```python
from build123d import *

# Parameters (mm, degrees)
F0_R          = 0.79375
F1_DEPTH      = 5.334
F3_DEPTH      = 5.334
F4_R          = 0.127
F5_W          = 2.54
F5_H          = 2.8669180299
F6_DEPTH      = 3.0408234879
F6_DEPTH_BACK = 0.8715074616
F7_SIZE       = 2.032


with BuildPart() as f1:
    # F0 (on Front) → F1 (new body)
    with BuildSketch(Plane.XZ):
        with BuildLine():
            ThreePointArc((-1.5158234879, 0.1576551724), (0, -1.524), (1.5158234879, 0.1576551724))
            Line((1.5158234879, 0.1576551724), (0.757911744, 7.4448275862))
            ThreePointArc((0.757911744, 7.4448275862), (0, 8.128), (-0.757911744, 7.4448275862))
            Line((-0.757911744, 7.4448275862), (-1.5158234879, 0.1576551724))
        make_face()
        Circle(F0_R, mode=Mode.SUBTRACT)
    extrude(amount=F1_DEPTH)

    # F2 (on face) → F3 (join, through all)
    with BuildSketch(Plane.XZ.offset(5.334)):
        Polygon((1.5158234879, 2.6129180299), (1.2631934914, 2.586642922), (1.5158234879, 0.1576551724), align=None)
        with BuildLine():
            Line((2.62023831, 4.4970114676), (0.6525069605, 7.7595462699))
            ThreePointArc((0.6525069605, 7.7595462699), (0.7225525537, 7.6079954691), (0.757911744, 7.4448275862))
            Line((0.757911744, 7.4448275862), (0.9662072397, 5.4421073456))
            Line((0.9662072397, 5.4421073456), (2.62023831, 4.4970114676))
        make_face()
    extrude(amount=-F3_DEPTH)

    # F4
    f4_edges = [f1.edges().sort_by_distance(p)[0] for p in [
        (2.620238, -2.667, 4.497011),
        (0.966207, -2.667, 5.442107),
    ]]
    fillet(f4_edges, radius=F4_R)

    # F5 (on face) → F6 (cut, two sides)
    with BuildSketch(Plane.YZ.offset(1.5158234879)) as f6_sk:
        with Locations((-2.667, -0.090540985)):
            Rectangle(F5_W, F5_H)
    extrude(amount=-F6_DEPTH, mode=Mode.SUBTRACT)
    extrude(f6_sk.sketch, amount=F6_DEPTH_BACK, mode=Mode.SUBTRACT)

    # F7
    f7_edges = [f1.edges().sort_by_distance(p)[0] for p in [
        (-1.392549, -2.667, 1.342918),
    ]]
    chamfer(f7_edges, length=F7_SIZE)


solid = f1.part
```
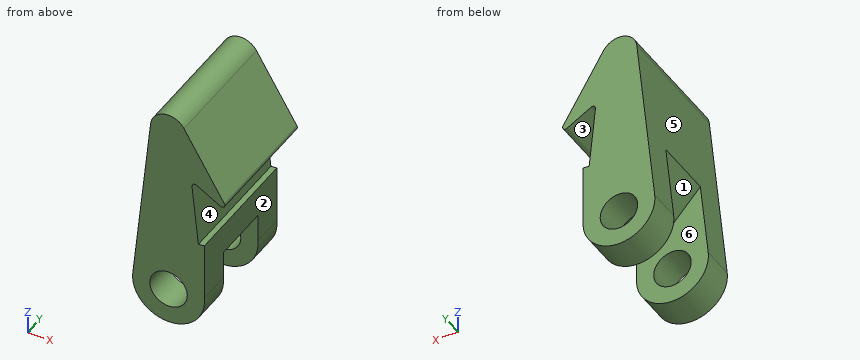
The model under review builds one solid part; all positions refer to its coordinate system, in mm. Face numbers are marked on the shaded views. A direction names the side the tool comes from. Coordinates: 2 decimals unless noted, no trailing zeros. Write each loop counter-clockwise with the first axis right and the second up, starting at its lowest first coordinate (ties: lowest second). Pieces come first, ordered by that corner, then holes. Notation, with made-up numbers: (28.25, 0) - (41.25, 0) arc R34 cw to (41.25, 37) - close; hole circle Ø2 at (89.25, -23.75). An arc over 180 degrees is marked (long way). Answer in a Markdown table with one row per item. Add a question column.
Q1. Consider section A-A on z = 0. Give the boundary of the cut face in (x, y).
Q2. For the marked faces 1, 2 and 3, list the 3-axis set-ups (+Z, -Z, +X, -X, +Y, -Y) from which the entire face can be reached by the end or side of a thin tool; tool diameter is ignored.
Q3. Consider section D-D on z = 1. Give the boundary of the cut face in (x, y), then the cut area to 3 significant figures.
Q4. Consider section B-B on x = 0.25. Give the boundary of the cut face in (y, z).
Q5. To check wall thickness, follow line 1 along X through (y, z) = (-0.6, 0); line 2 along Y through (x, z) = (1.4, 0.75); line 3 along Z through (x, y) = (2.2, -0.85). State the ranges of each line that lie inside material, in increasing order. Write a range as from..to.
Q6. Draft analysis for pull direction Z (two halves, no side actions). For the marked faces 4, 5 and 6, state which applies: +Z half, -Z half, draft (parallel to the pull), parting line (faces both ways), or undercut.
Q7. Clearance check with flat-ended pins moving along their axes: pin 1 (1 mm diameter, centred on x = 1, y = -2, fed in from -Z); pin 2 (2.5 mm diameter, centred on y = -3.5, z = 2, fed in from +X). State where each tip first meets the part, or that it passes through.
Answers below:
| question | item | result |
|---|---|---|
| 1 | outline | (-1.52, -5.33) - (-0.79, -5.33) - (-0.79, -3.94) - (-1.52, -3.94) - close; (-1.52, -1.4) - (-0.79, -1.4) - (-0.79, 0) - (-1.52, 0) - close; (0.79, -5.33) - (1.52, -5.33) - (1.52, -3.94) - (0.79, -3.94) - close; (0.79, -1.4) - (1.52, -1.4) - (1.52, 0) - (0.79, 0) - close |
| 2 | face 1 | -Z, -X |
| 2 | face 2 | +X, +Y, -Y |
| 2 | face 3 | +Y, -Y |
| 3 | outline | (-1.43, -5.33) - (1.52, -5.33) - (1.52, -3.94) - (-1.43, -3.94) - close; (-1.43, -1.4) - (1.52, -1.4) - (1.52, 0) - (-1.43, 0) - close |
| 3 | area | 8.23 mm² |
| 4 | outline | (-5.33, -1.5) - (-3.94, -1.5) - (-3.94, -0.75) - (-5.33, -0.75) - close; (-5.33, 0.75) - (-3.94, 0.75) - (-3.94, 1.77) - (-1.4, 1.77) - (-1.4, 0.75) - (0, 0.75) - (0, 8.09) - (-5.33, 8.09) - close; (-1.4, -1.5) - (0, -1.5) - (0, -0.75) - (-1.4, -0.75) - close |
| 5 | line 1 | -1.52..-0.79, 0.79..1.52 |
| 5 | line 2 | -5.33..-3.94, -1.4..0 |
| 5 | line 3 | 4.74..5.19 |
| 6 | face 4 | undercut |
| 6 | face 5 | +Z half |
| 6 | face 6 | draft |
| 7 | pin 1 | z = 1.34 |
| 7 | pin 2 | x = 1.52 |
